Read the model definition and answer for the solid it produces. Units are mm, in the model's axes. A direction names the side the tool comes from. Give positions to 0.01 mm unless a question says otherwise; leave off trailing zeros. Order: outer loops, then holes, each group sorted by start corner. A loop starts at its lowest first (then second) coordinate and runs counter-clockwise, first axis right, second up.
Item 1: Find the intervals of material crossed by line 1 along Z through (x, y) = (36.5, 13.25); line 2 along Z through (x, y) = (38.5, 1.25); line 3 along X through (y, z) = (9, -4.75), in increasing order.
Item 2: A cutting plane is placed at D-D (z = -8.5). Write down the section's boundary in (x, y).
Item 3: A cutting plane is placed at C-C (x = 3). Write down the section's boundary in (y, z), plus the area to 3 significant figures.
Item 4: A cutting plane is placed at A-A (z = -4.5). Write down the section's boundary in (x, y).
Item 5: A cutting plane is placed at B-B (y = 10). Write down the section's boundary in (x, z).
Item 6: The mould has two halves that part along X. Classify faces 6 (the face through (31, 8, -7)), 7 (the face through (3.39, 7.6, -6.91)), 8 (the face through (20, 15, -5)): +X half, -X half, draft (parallel to the pull), parting line (faces both ways), or undercut.
Item 7: Given pin 1 Ø2.5 at (x, y) = (37.5, 9) entering from -Z; pin 2 Ø0.5 at (y, z) = (9.5, -7) entering from -X; pin 3 Ø4 at (y, z) = (9, -2.5) entering from -X, each flat-ended and moving along its own axis, determine where each tip first touches the part or whether it passes through.
Item 8: Which of the six approach directions +Z, -Z, +X, -X, +Y, -Y give full straight-line access (tool end or side, diameter ignored) to faces 1 (the face through (36, 8, -6)), 2 (the face through (21, 7, -10)), 3 (the face through (34.071, 8, -7)), 4 (the face through (20, 7, 0)), 5 (the face through (37, 8, -8))?
from build123d import *

# Parameters (mm, degrees)
SKETCH1_W           = 40
SKETCH1_H           = 10
BOSS_EXTRUDE1_DEPTH = 15
CUT_EXTRUDE1_DEPTH  = 44.874821937
CUT_EXTRUDE2_DEPTH  = 44.874821937
CHAMFER1_SIZE       = 0.5


with BuildPart() as part:
    # Sketch1 → Boss-Extrude1 (new body)
    with BuildSketch(Plane(origin=(0, 0, 0), x_dir=(1, 0, 0), z_dir=(0, 1, 0))):
        with Locations((20, 5)):
            Rectangle(SKETCH1_W, SKETCH1_H)
    extrude(amount=BOSS_EXTRUDE1_DEPTH)

    # Sketch2 → Cut-Extrude1 (cut, through all)
    with BuildSketch(Plane(origin=(0, 15, 0), x_dir=(1, 0, 0), z_dir=(0, 1, 0))):
        with BuildLine():
            Line((10.663840824, 10), (0, 10))
            Line((0, 10), (0, 0))
            ThreePointArc((0, 0), (3.469314238, 6.986253576), (10.663840824, 10))
        make_face()
    extrude(amount=-CUT_EXTRUDE1_DEPTH, mode=Mode.SUBTRACT)

    # Sketch3 → Cut-Extrude2 (cut, through all)
    with BuildSketch(Plane(origin=(0, 15, 0), x_dir=(1, 0, 0), z_dir=(0, 1, 0))):
        Polygon((40, 10), (31, 10), (31, 4), (37, 4), (37, 6), (34.071499669, 6), (34.071499669, 8), (40, 8), align=None)
    extrude(amount=-CUT_EXTRUDE2_DEPTH, mode=Mode.SUBTRACT)

    # Chamfer1
    chamfer1_edges = [part.edges().sort_by_distance(p)[0] for p in [
        (34.071499669, 7.5, -8),
        (34.071499669, 7.5, -6),
    ]]
    chamfer(chamfer1_edges, length=CHAMFER1_SIZE)


solid = part.part
Response values:
1. line 1: z = -8 to -6, -4 to 0
1. line 2: z = -8 to 0
1. line 3: x = 1.63 to 31, 37 to 40
2. outline: (5.5, 0) - (31, 0) - (31, 15) - (5.5, 15) - close
3. outline: (0, -6.52) - (15, -6.52) - (15, 0) - (0, 0) - close
3. area: 97.8 mm2
4. outline: (1.48, 0) - (31, 0) - (31, 15) - (1.48, 15) - close; (37, 0) - (40, 0) - (40, 15) - (37, 15) - close
5. outline: (0, 0) arc R11.17 ccw to (10.66, -10) - (31, -10) - (31, -4) - (37, -4) - (37, -6) - (34.57, -6) - (34.07, -6.5) - (34.07, -7.5) - (34.57, -8) - (40, -8) - (40, 0) - close
6. face 6: undercut
6. face 7: -X half
6. face 8: draft
7. pin 1: stops at z = -8
7. pin 2: stops at x = 3.22
7. pin 3: stops at x = 0.06
8. face 1: +Y, -Y
8. face 2: -Z, +X, -X, +Y, -Y
8. face 3: -Z, +Y, -Y
8. face 4: +Z, +X, -X, +Y, -Y
8. face 5: -Z, +X, +Y, -Y
